Print and shaded views of the part. All mm, measured from the part's lowest x, y and z. Coordinates: 2 decimals unless noted, no trailing zeros. Loops run counter-clockwise (first coordinate to the right, second up) from the corner with the lowest first, then second, coordinate; pieces in that order, holes last.
1) Wall check: line 1 along X through (y, z) = (8.5, 1.15); line 2 along Y through (x, z) = (27, 0.6) (3 decimals); line 3 along X through (y, z) = (72, 3.2). Give the ranges that are in metal, low to high.
2) Saw through at B-B, the plane z = 2.2. Write the cut outline in (x, y).
3) Saw through at D-D, the plane x = 21. Write the cut outline in (y, z), and give its area (3 significant figures).
4) Saw through at C-C, the plane x = 27. Write the cut outline in (y, z) (3 decimals).
5) Two-plate mould, pull along X, no slides. Class the marked faces 1 and 2: +X half, -X half, draft (parallel to the pull), parting line (faces both ways), or undercut.
6) Saw through at A-A, the plane y = 10. Write the cut outline in (x, z).
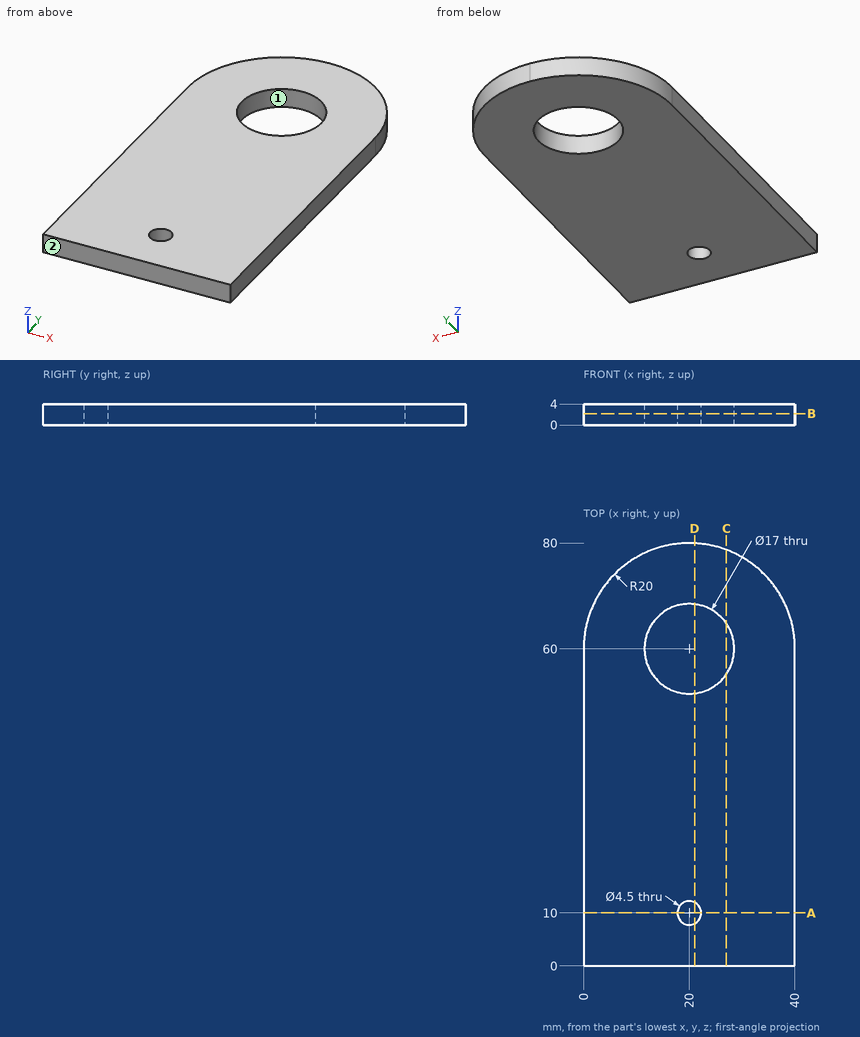
Data:
1. line 1: x = 0 to 18.32, 21.68 to 40
1. line 2: y = 0 to 55.178, 64.822 to 78.735
1. line 3: x = 4 to 36
2. outline: (0, 0) - (40, 0) - (40, 60) arc R20 ccw to (20, 80) arc R20 ccw to (0, 60) - close; hole circle Ø17 at (20, 60); hole circle Ø4.5 at (20, 10)
3. outline: (0, 0) - (7.98, 0) - (7.98, 4) - (0, 4) - close; (12.02, 0) - (51.56, 0) - (51.56, 4) - (12.02, 4) - close; (68.44, 0) - (79.97, 0) - (79.97, 4) - (68.44, 4) - close
3. area: 236 mm2
4. outline: (0, 0) - (55.178, 0) - (55.178, 4) - (0, 4) - close; (64.822, 0) - (78.735, 0) - (78.735, 4) - (64.822, 4) - close
5. face 1: undercut
5. face 2: draft
6. outline: (0, 0) - (17.75, 0) - (17.75, 4) - (0, 4) - close; (22.25, 0) - (40, 0) - (40, 4) - (22.25, 4) - close
